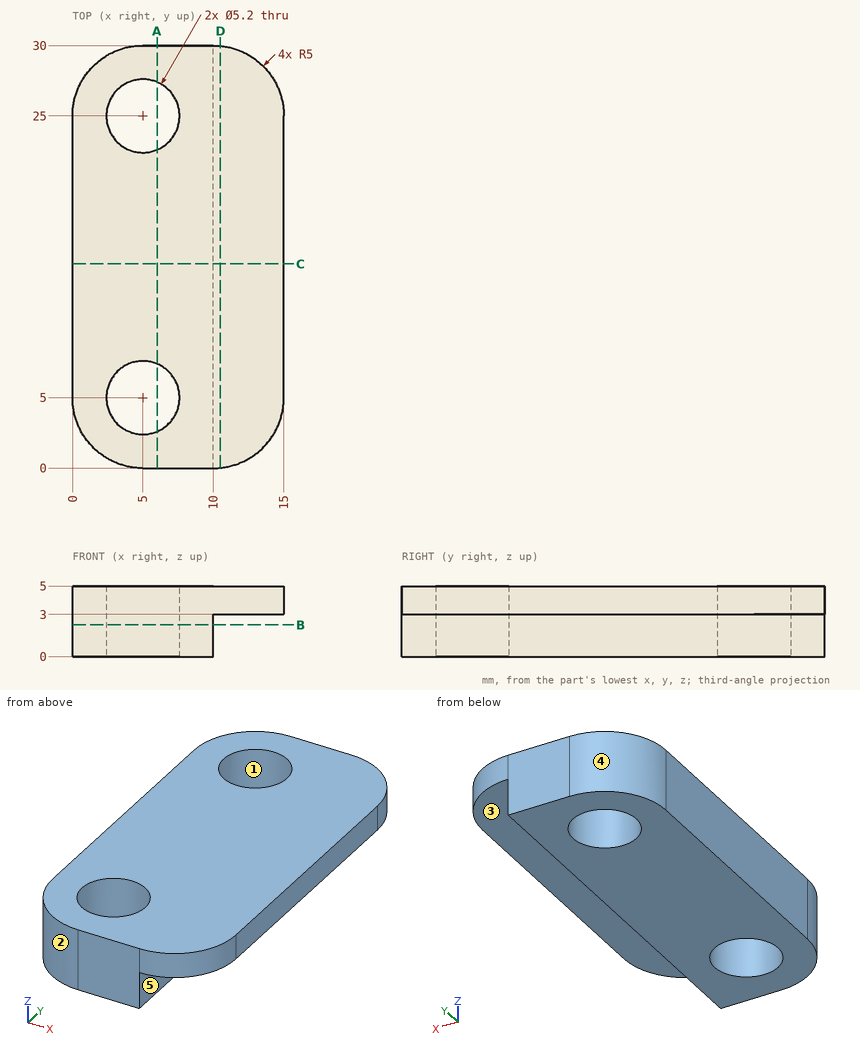
Here's the drawing with two shaded views (mm, measured from the low corner). I have some questions. A direction names the side the tool comes from. Coordinates: 2 decimals unless noted, no trailing zeros. Loops run counter-clockwise (first coordinate to the right, second up) from the corner with the lowest first, then second, coordinate; pieces in that order, holes last. Notation, with made-up numbers: (43.5, 43) -> (84.5, 43) arc R11 ccw to (84.5, 49) -> close; hole circle Ø5 at (79.5, 63.25). An arc over 180 degrees is marked (long way). Put each result on its own line as item: value. Start each with the question number.
Q1. I want a section at D-D (x = 10.5). Write out the boundary of the cut face in (y, z), plus the area to 3 significant figures.
Q2. If I drill on line 1 (Y direction, x = 5, z = 2.65); line 2 (Y direction, x = 4, z = 4); line 3 (X direction, y = 26.5, z = 2.25), over which ranges is the centre line in solid material (lowest first)? Write a range as [from, to].
Q3. I want a section at C-C (y = 14.5). Write out the boundary of the cut face in (x, z).
Q4. Thinking about a two-plate mould opening in Y: for the marked faces 1, 2 and 3, which applies, pulls with the +Y half, pulls with the -Y half, needs draft (parallel to the pull), parting line crosses it, or undercut?
Q5. For the marked faces 4 and 5, which set-ups out of +Z, -Z, +X, -X, +Y, -Y let a thin tool reach every point of the face, with its end or its side?
Q6. I'm going to push a flat-ended pin straight in: P1, Ø2.5, axis at x = 12.5, y = 20.5, coming from the -Z side. Where does the tip first touch, or does it pass through?
Q7. I want a section at B-B (z = 2.25). Write out the boundary of the cut face in (x, y).
Q8. I want a section at A-A (x = 6). Write out the boundary of the cut face in (y, z), plus the area to 3 significant figures.
Taken from the geometry:
1. outline: (0.03, 3) -> (29.97, 3) -> (29.97, 5) -> (0.03, 5) -> close
1. area: 59.9 mm2
2. line 1: y = [0, 2.4], [7.6, 22.4], [27.6, 30]
2. line 2: y = [0.1, 2.6], [7.4, 22.6], [27.4, 29.9]
2. line 3: x = [0.23, 2.88], [7.12, 10]
3. outline: (0, 0) -> (10, 0) -> (10, 3) -> (15, 3) -> (15, 5) -> (0, 5) -> close
4. face 1: undercut
4. face 2: pulls with the -Y half
4. face 3: needs draft
5. face 4: +Z, -Z, -X, +Y
5. face 5: -Z, +X, +Y, -Y
6. P1: stops at z = 3
7. outline: (0, 5) arc R5 ccw to (5, 0) -> (10, 0) -> (10, 30) -> (5, 30) arc R5 ccw to (0, 25) -> close; hole circle Ø5.2 at (5, 5); hole circle Ø5.2 at (5, 25)
8. outline: (0, 0) -> (2.6, 0) -> (2.6, 5) -> (0, 5) -> close; (7.4, 0) -> (22.6, 0) -> (22.6, 5) -> (7.4, 5) -> close; (27.4, 0) -> (30, 0) -> (30, 5) -> (27.4, 5) -> close
8. area: 102 mm2
